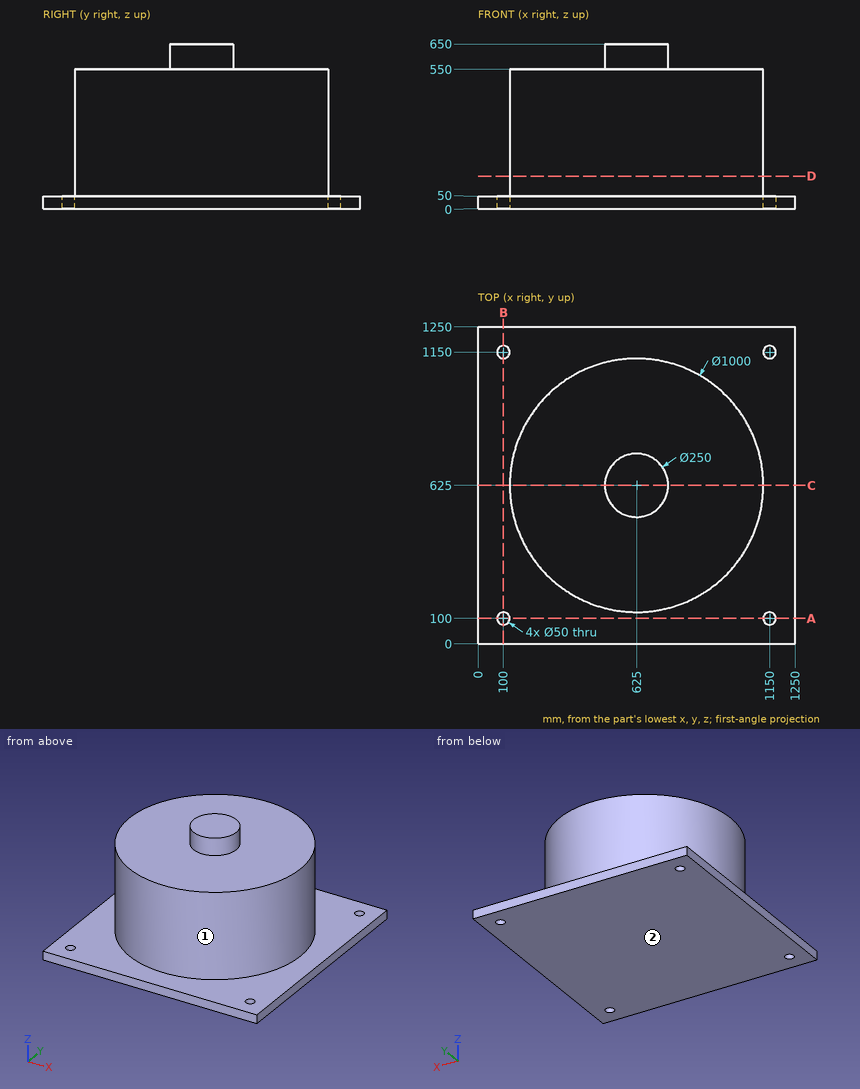
Could you check a few things on this drawing? It's one solid part, dimensions in mm from its lowest x, y, z. A direction names the side the tool comes from. Coordinates: 2 decimals unless noted, no trailing zeros. Write each loop counter-clockwise with the first axis right and the second up, starting at its lowest first coordinate (ties: lowest second). Pieces come first, ordered by that corner, then holes. Notation, with made-up numbers: (-11, 43) - (45, 43) arc R27 ccw to (45, 72) - close; hole circle Ø9 at (8.25, 80.25). An arc over 180 degrees is marked (long way). Put each result on its own line as item: value. Start each with the question number.
Q1. I want a section at C-C on y = 625. Write out the boundary of the cut face in (x, z), plus the area to 4 significant figures.
Q2. I want a section at A-A on y = 100. Write out the boundary of the cut face in (x, z).
Q3. I want a section at D-D on z = 129. Write out the boundary of the cut face in (x, y).
Q4. Please list where these lines run through material, in increasing order: L1, parallel to X at y = 1150, z = 22; L2, parallel to Z at x = 236.5, y = 369.5.
Q5. I'm going to push flat-ended pins straight in: P1, Ø5, axis at y = 1072.5, z = 517.5, coming from the -X side; P2, Ø3, axis at x = 218.5, y = 659, coming from the +Z side; P3, Ø2, axis at x = 800, z = 493, coming from the -Y side. Where does each tip first touch, or does it pass through?
Q6. Which directions (+Z, -Z, +X, -X, +Y, -Y) give clear straight access to the entire face, cutting with the end or side of a thin tool? Please do the marked faces 1 and 2.
Checks:
1. outline: (0, 0) - (1250, 0) - (1250, 50) - (1125, 50) - (1125, 550) - (750, 550) - (750, 650) - (500, 650) - (500, 550) - (125, 550) - (125, 50) - (0, 50) - close
1. area: 587,500 mm²
2. outline: (0, 0) - (75, 0) - (75, 50) - (0, 50) - close; (125, 0) - (1125, 0) - (1125, 50) - (125, 50) - close; (1175, 0) - (1250, 0) - (1250, 50) - (1175, 50) - close
3. outline: circle Ø1000 at (625, 625)
4. L1: 0 to 75, 125 to 1125, 1175 to 1250
4. L2: 0 to 550
5. P1: x = 397.02
5. P2: z = 550
5. P3: y = 156.25
6. face 1: +Z
6. face 2: -Z, +X, -X, +Y, -Y
